Read the model definition and answer for the solid it produces. Units are mm, in the model's axes. A direction names the side the tool comes from. Give positions to 0.01 mm unless a question says otherwise; leave off trailing zeros. Order: outer loops, then holes, each group sorted by start corner. A loop starts at its lowest first (then second) coordinate and runs counter-clockwise, first axis right, second up. Notation, with made-up numbers: (-31.75, 36.25) -> (-21.75, 36.25) arc R30 ccw to (-21.75, 58.25) -> close; hole circle Ø4 at (9.5, 0.5). An arc over 180 degrees is marked (long way). Answer as CSV lines item,"result". Start each with the question number.
1) The mould has two halves that part along Y. Classify faces 1 (the face through (270, 215.9, 457)), 2 (the face through (277, 476.25, 457)), 3 (the face through (50.8, 100, 25)), 4 (the face through (495.3, 257, 25)): +Y half, -Y half, draft (parallel to the pull), parting line (faces both ways), or undercut.
2) Straight lines are drawn through the part: L1, parallel to Y at x = 273, z = 137.5; L2, parallel to X at y = 335.5, z = 854.5; L3, parallel to Z at x = 49.5, y = 195. For each, find the intervals that lie inside material, in ascending order. Write a range as from..to.
3) Find section A-A (x = 250.5). Determine the outline of the cut face in (y, z).
4) Find section B-B (y = 110). Determine the outline of the cut face in (x, z).
5) Find section C-C (z = 655.5). Determine the outline of the cut face in (x, y).
6) For faces 5 (the face through (521, 210, 50.384)), 6 (the face through (495.3, 100, 877)), 7 (the face through (50.8, 319, 25)), determine the directions among +Z, -Z, +X, -X, +Y, -Y from which every point of the face is accessible in a straight line to the end or side of a thin tool.
7) Flat-ended cylindrical pins translate along their axes: pin 1 Ø4 at (x, z) = (268, 282) entering from -Y; pin 2 Ø4 at (y, z) = (209, 619.5) entering from -X; pin 3 Ø15 at (x, y) = (20, 120) entering from -Z. Find the tip coordinate at first contact, or state that the pin passes through.
Autodesk Fusion 360 part; units mm, degrees
sketch "Sketch1" plane through (0, 0, 0) normal (0, 1, 0) x (1, 0, 0)
  line L0 (0, 0) -> (50.8, 0)
  line L1 (50.8, 0) -> (50.8, -50.8)
  line L2 (50.8, -50.8) -> (0, -50.8)
  line L3 (0, -50.8) -> (0, 0)
  line L4 (0, -850.9) -> (50.8, -850.9)
  line L5 (50.8, -850.9) -> (50.8, -901.7)
  line L6 (50.8, -901.7) -> (0, -901.7)
  line L7 (0, -901.7) -> (0, -850.9)
  line L8 (0, -50.8) -> (0, 0)
  line L9 (50.8, 0) -> (50.8, -50.8)
  line L10 (0, 0) -> (50.8, 0)
  line L11 (50.8, -50.8) -> (0, -50.8)
  line L12 (546.1, -50.3836) -> (495.3, -50.3836)
  line L13 (546.1, 0.4164) -> (546.1, -50.3836)
  line L14 (495.3, 0.4164) -> (546.1, 0.4164)
  line L15 (495.3, -50.3836) -> (495.3, 0.4164)
  line L16 (495.3, -850.9) -> (546.1, -850.9)
  line L17 (546.1, -850.9) -> (546.1, -901.7)
  line L18 (546.1, -901.7) -> (495.3, -901.7)
  line L19 (495.3, -901.7) -> (495.3, -850.9)
  dimension "d1" = 50.8
  dimension "d2" = 50.8
  dimension "d3" = 50.8
  dimension "d4" = 50.8
  dimension "d5" = 800.1
  dimension "d6" = 50.8
  dimension "d7" = 50.8
  dimension "d8" = 50.8
  dimension "d9" = 50.8
  dimension "d10" = 444.5
  dimension "d11" = 50.8
  dimension "d12" = 50.8
extrude "Extrude1" add sketch "Sketch1" along normal blind 425.45 makes body 1 at (512.2333, 141.8167, 850.9) makes body 2 at (529.1667, 141.8167, 50.3836) makes body 3 at (16.9333, 141.8167, 850.9) makes body 4 at (16.9333, 141.8167, 0)
sketch "Sketch2" plane through (0, 425.45, 0) normal (0, 1, 0) x (-1, 0, 0)
  line L0 (0, 901.7) -> (-50.8, 901.7)
  line L1 (-50.8, 901.7) -> (-50.8, 850.9)
  line L2 (-50.8, 850.9) -> (0, 850.9)
  line L3 (0, 850.9) -> (0, 901.7)
  line L4 (0, 901.7) -> (-546.1, 901.7)
  line L5 (-546.1, 901.7) -> (-546.1, -0.4164)
  line L6 (-546.1, -0.4164) -> (0, -0.4164)
  line L7 (0, -0.4164) -> (0, 901.7)
  point P0 (-546.1, -0.4164)
extrude "Extrude2" add sketch "Sketch2" along normal blind 50.8 bodies 1 2 3 4
sketch "Sketch3" plane through (0, 0, 901.7) normal (0, 0, 1) x (1, 0, 0)
  line L0 (495.3, 0) -> (546.1, 0)
  line L1 (546.1, 0) -> (546.1, 476.25)
  line L2 (546.1, 476.25) -> (0, 476.25)
  line L3 (0, 476.25) -> (0, 0)
  line L4 (0, 0) -> (50.8, 0)
  line L5 (50.8, 0) -> (50.8, 425.45)
  line L6 (50.8, 425.45) -> (495.3, 425.45)
  line L7 (495.3, 425.45) -> (495.3, 0)
  line L8 (50.8, 215.9) -> (495.3, 215.9)
  line L9 (495.3, 215.9) -> (495.3, 203.2)
  line L10 (495.3, 203.2) -> (50.8, 203.2)
  line L11 (50.8, 203.2) -> (50.8, 215.9)
  dimension "d22" = 444.5
  dimension "d23" = 12.7
  dimension "d24" = 203.2
extrude "Extrude3" add sketch "Sketch3" against normal blind 901.7 contours L5 L7 L8 L9 L10 L11 bodies 1
Findings below:
1,face 1,"undercut"
1,face 2,"+Y half"
1,face 3,"draft"
1,face 4,"undercut"
2,L1,"203.2..215.9, 425.45..476.25"
2,L2,"0..50.8, 495.3..546.1"
2,L3,"0..50.8, 850.9..901.7"
3,outline,"(203.2, 0) -> (215.9, 0) -> (215.9, 901.7) -> (203.2, 901.7) -> close; (425.45, -0.42) -> (476.25, -0.42) -> (476.25, 901.7) -> (425.45, 901.7) -> close"
4,outline,"(0, 0) -> (50.8, 0) -> (50.8, 50.8) -> (0, 50.8) -> close; (0, 850.9) -> (50.8, 850.9) -> (50.8, 901.7) -> (0, 901.7) -> close; (495.3, -0.42) -> (546.1, -0.42) -> (546.1, 50.38) -> (495.3, 50.38) -> close; (495.3, 850.9) -> (546.1, 850.9) -> (546.1, 901.7) -> (495.3, 901.7) -> close"
5,outline,"(0, 425.45) -> (546.1, 425.45) -> (546.1, 476.25) -> (0, 476.25) -> close; (50.8, 203.2) -> (495.3, 203.2) -> (495.3, 215.9) -> (50.8, 215.9) -> close"
6,face 5,"+X, -Y"
6,face 6,"+Z, -Z, -Y"
6,face 7,"+Z, -Z"
7,pin 1,"y = 203.2"
7,pin 2,"x = 50.8"
7,pin 3,"z = 0"
